```python
from build123d import *

# Parameters (mm, degrees)
F0_W     = 64.6176
F0_H     = 19.05
F2_R     = 6.35
F3_DEPTH = 7.62
F4_R     = 3.81
F5_DEPTH = 33.02


with BuildPart() as f1:
    # F0 (on Front) → F1 (revolve)
    with BuildSketch(Plane.XZ):
        with Locations((6.097645, 9.525)):
            Rectangle(F0_W, F0_H)
    revolve(axis=Axis((6.097645, 0, 0), (1, 0, 0)))

    # F2 (on face) → F3 (join)
    with BuildSketch(Plane(origin=(-26.211155, 0, 0), x_dir=(0, -1, 0), z_dir=(-1, 0, 0))):
        with Locations((0, 8.60392)):
            Circle(F2_R)
    extrude(amount=F3_DEPTH)

    # F4 (on face) → F5 (join)
    with BuildSketch(Plane(origin=(-33.831155, 0, 0), x_dir=(0, -1, 0), z_dir=(-1, 0, 0))):
        with Locations((0, 8.60392)):
            Circle(F4_R)
    extrude(amount=F5_DEPTH)


solid = f1.part
```
Geometry check sheet. Reference: the model listing, model coordinates, mm. A direction names the side the tool comes from. Give positions to 0.01 mm unless a question says otherwise; leave off trailing zeros. Order: outer loops, then holes, each group sorted by start corner. A loop starts at its lowest first (then second) coordinate and runs counter-clockwise, first axis right, second up. Notation, with made-up numbers: (21, 53.5) -> (45, 53.5) arc R31 cw to (45, 85.5) -> close; hole circle Ø2 at (10.5, 29). An arc over 180 degrees is marked (long way). Write each question's results on one line, items separated by ' | '. Start each with the question number.
(1) Sectioned sample at B-B (x = -6.5). Enter the section's corners in (y, z), plus the area to 3 significant figures.
(2) Sectioned sample at D-D (x = -41). Enter the section's corners in (y, z), plus the area to 3 significant figures.
(3) Sectioned sample at C-C (z = 0). Enter the section's corners in (x, y), plus the area to 3 significant figures.
(4) Sectioned sample at A-A (y = 0). Enter the section's corners in (x, z), plus the area to 3 significant figures.
(5) Scan lines: line 1 (Y direction, x = -28.5, z = 8.5); line 2 (X direction, y = -8, z = -12.5); line 3 (X direction, y = 1.5, z = 4). Record each from-to range of solid material in increasing order.
(6) Gauge pin test, flat ends, axial feed: P1, Ø19, axis at y = 8, z = 3.5, coming from the -X side; P2, Ø1.5, axis at x = 25, z = -1.5, coming from the -Y side; P3, Ø4, axis at y = -14, z = 10, coming from the -X side; P4, Ø10, axis at x = 14.5, z = 9, coming from the -Y side. Record the tip position at first contact, or that the pin passes through.
(7) Access from +Z, -Z, +X, -X, +Y, -Y to the whole of each face (thin tool, end or side, straight path). Record for faces 1 (the face through (-33.831, -3, 6)), 2 (the face through (38.406, 0, 0)).
Answer below:
1) outline: circle Ø38.1 at (0, 0) | area: 1,140 mm2
2) outline: circle Ø7.62 at (0, 8.6) | area: 45.6 mm2
3) outline: (-26.21, -19.05) -> (38.41, -19.05) -> (38.41, 19.05) -> (-26.21, 19.05) -> close | area: 2,460 mm2
4) outline: (-66.85, 4.79) -> (-33.83, 4.79) -> (-33.83, 2.25) -> (-26.21, 2.25) -> (-26.21, -19.05) -> (38.41, -19.05) -> (38.41, 19.05) -> (-26.21, 19.05) -> (-26.21, 14.95) -> (-33.83, 14.95) -> (-33.83, 12.41) -> (-66.85, 12.41) -> close | area: 2,810 mm2
5) line 1: -6.35 to 6.35 | line 2: -26.21 to 38.41 | line 3: -33.83 to 38.41
6) P1: x = -66.85 | P2: y = -19.04 | P3: x = -26.21 | P4: y = -18.63
7) face 1: -X | face 2: +Z, -Z, +X, +Y, -Y
